Read the model definition and answer for the solid it produces. Units are mm, in the model's axes. Round coordinates to 2 decimals unless told otherwise and drop trailing zeros. Order: outer loops, then holes, each group sorted by start corner. A loop starts at its lowest first (then second) coordinate and runs counter-clockwise, first axis right, second up. Notation, with made-up numbers: (-2.75, 30.5) -> (20.25, 30.5) arc R27 ccw to (20.25, 55.5) -> close; hole circle Ø3 at (53.5, 62). An arc over 180 degrees is marked (long way). Use a Markdown table: item, result. Add a question column.
1. Section C-C, the plane x = -31 is taken. Give the vertices of the cut face in (y, z).
2. Given pin 1 (10 mm diameter, centred on x = -22, z = 20.5, fed in from -Y); pin 2 (1.5 mm diameter, centred on x = -48, z = 24, fed in from -Y); pin 3 (4 mm diameter, centred on x = -13, z = 13.5, fed in from -Y); pin 4 (6 mm diameter, centred on x = -50.5, y = 54, fed in from +Z), each flat-ended and moving along its own axis, determine where each tip first touches the part or whether it passes through.
3. Consider L1, parallel to Y at x = 0, z = 26.75; L2, parallel to Y at x = -20, z = 28.25; L3, parallel to X at y = 49.5, z = 11. Determine where each line is inside the solid, lowest interval first. Write a range as [from, to].
4. Section A-A, the plane z = 27 is taken. Give the vertices of the cut face in (x, y).
5. Section B-B, the plane y = 54 is taken. Give the vertices of the cut face in (x, z).
Autodesk Inventor part; units mm, degrees
ref_plane "YZ Plane" through (0, 0, 0) normal (1, 0, 0) x (0, 1, 0)
ref_plane "XZ Plane" through (0, 0, 0) normal (0, 1, 0) x (-1, 0, 0)
ref_plane "XY Plane" through (0, 0, 0) normal (0, 0, 1) x (1, 0, 0)
sketch "スケッチ1" plane through (0, 0, 0) normal (0, 0, 1) x (1, 0, 0)
  circle A0 centre (-56.2051, 45.5451) radius 2.75
  arc A1 (8.9566, 76.3281) -> (6.09, 76.7004) centre (7.222, 74.1942) ccw
  circle A2 centre (57.2805, 33.1812) radius 3
  line L0 (-57.3371, 48.0513) -> (6.09, 76.7004)
  line L1 (8.9566, 76.3281) -> (59.1728, 35.5091)
  line L2 (-57.543, 48.5069) -> (5.8841, 77.1561)
  arc A3 (6.09, 76.7004) -> (8.9566, 76.3281) centre (7.222, 74.1942) ccw
  arc A4 (9.4296, 76.9101) -> (5.7812, 77.3839) centre (7.222, 74.1942) ccw
  line L3 (9.4296, 76.9101) -> (59.6459, 36.0911)
  line L4 (-57.543, 48.5069) -> (-56.2051, 45.5451)
  line L5 (57.2805, 33.1812) -> (59.6459, 36.0911)
  line L6 (-52.9862, 50.5651) -> (-52.7804, 50.1095)
  line L7 (55.2929, 38.663) -> (55.766, 39.2449)
  line L8 (5.7812, 77.3839) -> (7.222, 74.1942)
  line L9 (1.3274, 75.0979) -> (1.5332, 74.6422)
  point P0 (0, 0)
  point P1 (5.7812, 77.3839)
  point P2 (6.09, 76.7004)
  point P3 (5.8841, 77.1561)
  dimension "d0" = 0.5
  dimension "d1" = 0.75
  dimension "d2" = 0.75
  dimension "d3" = 5
  dimension "d4" = 5
  dimension "d17" = 5
extrude "押し出し1" add sketch "スケッチ1" along normal blind 30 contours L4 L2 L6 L0 | L6 L2 L9 L0 | L9 L2 L8 L0
sketch "スケッチ2" plane through (-57.543, 48.5069, 30) normal (-0.4116, 0.9113, 0) x (0.9113, 0.4116, 0)
  line L0 (69.5972, 30) -> (0, 30)
  line L1 (0, 30) -> (0, 0)
  line L2 (69.5972, 0) -> (0, 0)
  circle A0 centre (5, 15) radius 1.5
  line L3 (69.5972, 30) -> (69.5972, 0)
  circle A1 centre (64.5972, 15) radius 1.5
  point P0 (32.474, 30)
  dimension "d7" = 3
  dimension "d8" = 15
  dimension "d9" = 5
  dimension "d18" = 3
  dimension "d19" = 15
  dimension "d20" = 5
extrude "押し出し2" cut sketch "スケッチ2" against normal blind 0.75 contours A0 | A1
properties part number "クランクガード前" material "ポリカーボネート、クリア"
Verdict:
| question | item | result |
|---|---|---|
| 1 | outline | (59.95, 0) -> (60.5, 0) -> (60.5, 30) -> (59.95, 30) -> close |
| 2 | pin 1 | stops at y = 61.75 |
| 2 | pin 2 | stops at y = 51.93 |
| 2 | pin 3 | stops at y = 67.17 |
| 2 | pin 4 | stops at z = 30 |
| 3 | L1 | y = [73.95, 74.5] |
| 3 | L2 | y = [64.92, 65.46] |
| 3 | L3 | x = [-55.34, -54.13] |
| 4 | outline | (-57.54, 48.51) -> (-57.34, 48.05) -> (6.09, 76.7) -> (5.88, 77.16) -> close |
| 5 | outline | (-45.38, 0) -> (-44.17, 0) -> (-44.17, 30) -> (-45.38, 30) -> close |
